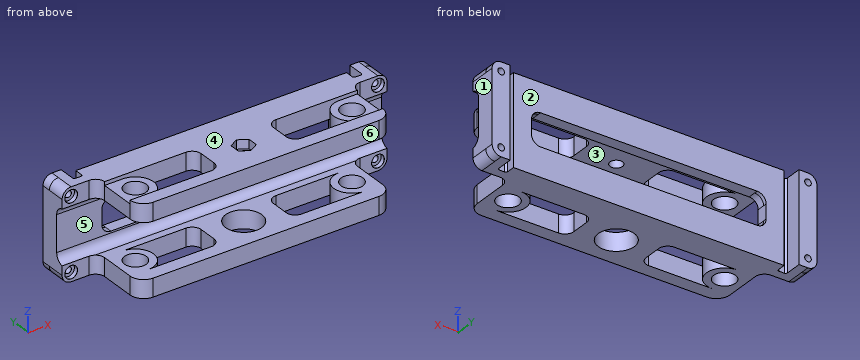
```python
from build123d import *

# Parameters (mm, degrees)
SKETCH_1_W                 = 150
SKETCH_1_H                 = 50
EXTRUDE_1_DEPTH            = 10
CUT_EXTRUDE_5_DEPTH        = 5
SKETCH_6_R                 = 6.05
CUT_EXTRUDE_6_DEPTH        = 80.686887253
CUT_EXTRUDE_7_DEPTH        = 80.686887253
CUT_EXTRUDE_8_DEPTH        = 80.686887253
SKETCH_9_R                 = 3.5
CUT_EXTRUDE_9_DEPTH        = 80.214897721
SKETCH_10_W                = 150
SKETCH_10_H                = 1.5
CUT_EXTRUDE_10_DEPTH       = 80.686887391
SKETCH_11_W                = 150
SKETCH_11_H                = 4.25
EXTRUDE_3_DEPTH            = 15
CUT_EXTRUDE_12_REACH       = 95.152
SKETCH_14_R                = 10
SKETCH_15_W                = 130
SKETCH_15_H                = 18
CUT_EXTRUDE_13_DEPTH       = 93.604333216
FILLET_1_R                 = 5
EXTRUDE_4_DEPTH            = 15
EXTRUDE_5_DEPTH            = 15
FILLET_2_R                 = 5
HOLE_WIZARD_M31_AT_2_COUNT = 2
HOLE_WIZARD_M31_AT_2_PITCH = 40
HOLE_WIZARD_M31_AT_3_COUNT = 2
HOLE_WIZARD_M31_AT_3_PITCH = 170
HOLE_WIZARD_M31_AT_4_COUNT = 2
HOLE_WIZARD_M31_AT_4_PITCH = 174.642491966
CUT_EXTRUDE_20_DEPTH       = 2
SKETCH_22_W                = 5
SKETCH_22_H                = 50
CUT_EXTRUDE_21_DEPTH       = 5
FILLET_3_R                 = 1
FILLET_4_R                 = 5
EXTRUDE_START              = 5
SKETCH_23_R                = 1.825
EXTRUDE_7_DEPTH            = 5
EXTRUDE_START_2            = 2
SKETCH_24_W                = 150
SKETCH_24_H                = 50
EXTRUDE_8_DEPTH            = 2


with BuildPart() as part:
    # Эскиз1 → Бобышка-Вытянуть1 (new body)
    with BuildSketch(Plane.XY):
        Rectangle(SKETCH_1_W, SKETCH_1_H)
    extrude(amount=EXTRUDE_1_DEPTH)

    # Эскиз5 → Вырез-Вытянуть5 (cut)
    with BuildSketch(Plane.XY.offset(10)):
        Polygon((0, 5.75), (-4.979646072, 2.875), (-4.979646072, -2.875), (0, -5.75), (4.979646072, -2.875), (4.979646072, 2.875), align=None)
    extrude(amount=-CUT_EXTRUDE_5_DEPTH, mode=Mode.SUBTRACT)

    # Эскиз6 → Вырез-Вытянуть6 (cut, through all)
    with BuildSketch(Plane.XY.offset(10)):
        with Locations((-60, 0)):
            Circle(SKETCH_6_R)
        with Locations(Location((60, 0, 0), (0, 0, 180))):
            Circle(SKETCH_6_R)
    extrude(amount=-CUT_EXTRUDE_6_DEPTH, mode=Mode.SUBTRACT)

    # Эскиз7 → Вырез-Вытянуть7 (cut, through all)
    with BuildSketch(Plane.XY.offset(10)):
        with BuildLine():
            Line((65, -25), (75, -25))
            Line((75, -25), (75, -15))
            Line((75, -15), (75, 15))
            ThreePointArc((75, 15), (71.464466094, 13.535533906), (70, 10))
            Line((70, 10), (70, -10))
            ThreePointArc((70, -10), (67.803300859, -15.303300859), (62.5, -17.5))
            Line((62.5, -17.5), (27.5, -17.5))
            Line((27.5, -17.5), (-2.5, -17.5))
            Line((-2.5, -17.5), (-32.5, -17.5))
            Line((-32.5, -17.5), (-62.5, -17.5))
            ThreePointArc((-62.5, -17.5), (-67.803300859, -15.303300859), (-70, -10))
            Line((-70, -10), (-70, 10))
            ThreePointArc((-70, 10), (-71.464466094, 13.535533906), (-75, 15))
            Line((-75, 15), (-75, -15))
            Line((-75, -15), (-75, -25))
            Line((-75, -25), (-65, -25))
            Line((-65, -25), (-25, -25))
            Line((-25, -25), (25, -25))
            Line((25, -25), (65, -25))
        make_face()
    extrude(amount=-CUT_EXTRUDE_7_DEPTH, mode=Mode.SUBTRACT)

    # Эскиз8 → Вырез-Вытянуть8 (cut, through all)
    with BuildSketch(Plane(origin=(0, 0, 0), x_dir=(-1, 0, 0), z_dir=(0, 0, -1))):
        with BuildLine():
            Line((20, -5), (20, 5))
            ThreePointArc((20, 5), (21.464466094, 8.535533906), (25, 10))
            Line((25, 10), (45, 10))
            add(Edge.make_bspline(
                [(60, 10), (59.955521003, 10), (54.127943117, 10), (45, 10)],
                knots=[0, 0, 0, 0, 1, 1, 1, 1], degree=3))
            ThreePointArc((60, 10), (50, 0), (60, -10))
            add(Edge.make_bspline(
                [(60, -10), (59.955521003, -10), (54.127943117, -10), (45, -10)],
                knots=[0, 0, 0, 0, 1, 1, 1, 1], degree=3))
            Line((45, -10), (25, -10))
            ThreePointArc((25, -10), (21.464466094, -8.535533906), (20, -5))
        make_face()
        with BuildLine():
            Line((-45, -10), (-25, -10))
            ThreePointArc((-25, -10), (-21.464466094, -8.535533906), (-20, -5))
            Line((-20, -5), (-20, 5))
            ThreePointArc((-20, 5), (-21.464466094, 8.535533906), (-25, 10))
            Line((-25, 10), (-45, 10))
            add(Edge.make_bspline(
                [(-60, 10), (-59.955521003, 10), (-54.127943117, 10), (-45, 10)],
                knots=[0, 0, 0, 0, 1, 1, 1, 1], degree=3))
            ThreePointArc((-60, 10), (-50, 0), (-60, -10))
            add(Edge.make_bspline(
                [(-60, -10), (-59.955521003, -10), (-54.127943117, -10), (-45, -10)],
                knots=[0, 0, 0, 0, 1, 1, 1, 1], degree=3))
        make_face()
    extrude(amount=-CUT_EXTRUDE_8_DEPTH, mode=Mode.SUBTRACT)

    # Эскиз9 → Вырез-Вытянуть9 (cut, through all)
    with BuildSketch(Plane.XY.offset(5)):
        Circle(SKETCH_9_R)
    extrude(amount=-CUT_EXTRUDE_9_DEPTH, mode=Mode.SUBTRACT)

    # Эскиз10 → Вырез-Вытянуть10 (cut, through all)
    with BuildSketch(Plane.XY.offset(10)):
        with Locations((0, 24.25)):
            Rectangle(SKETCH_10_W, SKETCH_10_H)
    extrude(amount=-CUT_EXTRUDE_10_DEPTH, mode=Mode.SUBTRACT)

    # Эскиз11 → Бобышка-Вытянуть3 (add)
    with BuildSketch(Plane(origin=(0, 0, 0), x_dir=(-1, 0, 0), z_dir=(0, 0, -1))):
        with Locations((0, 21.375)):
            Rectangle(SKETCH_11_W, SKETCH_11_H)
    extrude(amount=EXTRUDE_3_DEPTH)

    # Зеркальное отражение9: part across plane


with BuildPart() as part_1:
    add(part.part)
    add(part.part.mirror(Plane(origin=(0, 0, -15), x_dir=(1, 0, 0), z_dir=(0, 0, -1))))

    # Эскиз14 → Вырез-Вытянуть12 (cut, up to next)
    with BuildSketch(Plane(origin=(0, 0, -40), x_dir=(-1, 0, 0), z_dir=(0, 0, -1)), mode=Mode.PRIVATE) as cut_extrude_12_sk1:
        Circle(SKETCH_14_R)
    cut_extrude_12_tool1 = extrude(cut_extrude_12_sk1.sketch, amount=-CUT_EXTRUDE_12_REACH, mode=Mode.PRIVATE) & part_1.part
    add(cut_extrude_12_tool1.solids().sort_by_distance((0, 0, -40))[0], mode=Mode.SUBTRACT)

    # Эскиз15 → Вырез-Вытянуть13 (cut, through all)
    with BuildSketch(Plane.XZ.offset(-19.25)):
        with Locations((0, -15)):
            Rectangle(SKETCH_15_W, SKETCH_15_H)
    extrude(amount=-CUT_EXTRUDE_13_DEPTH, mode=Mode.SUBTRACT)

    # Скругление1
    fillet_1_edges = [part_1.edges().sort_by_distance(p)[0] for p in [
        (65, 21.375, -6),
        (65, 21.375, -24),
        (-65, 21.375, -24),
        (-65, 21.375, -6),
    ]]
    fillet(fillet_1_edges, radius=FILLET_1_R)

    # Эскиз18 → Бобышка-Вытянуть4 (add)
    with BuildSketch(Plane(origin=(75, 0, 0), x_dir=(0, 0, -1), z_dir=(1, 0, 0))):
        Polygon((-10, 23.5), (-10, 15), (0, 15), (0, 19.25), (30, 19.25), (30, 15), (40, 15), (40, 25), (-10, 25), align=None)
    extrude(amount=EXTRUDE_4_DEPTH)

    # Эскиз19 → Бобышка-Вытянуть5 (add)
    with BuildSketch(Plane.ZY.offset(75)):
        Polygon((-40, 15), (-30, 15), (-30, 19.25), (0, 19.25), (0, 15), (10, 15), (10, 25), (-40, 25), align=None)
    extrude(amount=EXTRUDE_5_DEPTH)

    # Скругление2
    fillet_2_edges = [part_1.edges().sort_by_distance(p)[0] for p in [
        (90, 20, 10),
        (90, 20, -40),
        (-90, 20, -40),
        (-90, 20, 10),
    ]]
    fillet(fillet_2_edges, radius=FILLET_2_R)

    # Эскиз20 → Цековка для винта с заклепочной головкой M31 (revolve, cut)
    with BuildSketch(Plane(origin=(-85, 15, -35), x_dir=(0, 0, -1), z_dir=(1, 0, 0))):
        Polygon((0, 0), (0, 10), (1.825, 10), (1.8, 9.975), (1.8, 2.425), (1.825, 2.4), (3.5, 2.4), (3.5, 0.025), (3.525, 0), align=None)
    hole_wizard_m31 = revolve(axis=Axis((-85, 8.65, -35), (0, 1, 0)), mode=Mode.SUBTRACT)

    # Цековка для винта с заклепочной головкой M31 at 2: Цековка для винта с заклепочной головкой M31 ×2
    with Locations(*[(0, 0, i * HOLE_WIZARD_M31_AT_2_PITCH) for i in range(1, HOLE_WIZARD_M31_AT_2_COUNT)]):
        add(hole_wizard_m31, mode=Mode.SUBTRACT)

    # Цековка для винта с заклепочной головкой M31 at 3: Цековка для винта с заклепочной головкой M31 ×2
    with Locations(*[(i * HOLE_WIZARD_M31_AT_3_PITCH, 0, 0) for i in range(1, HOLE_WIZARD_M31_AT_3_COUNT)]):
        add(hole_wizard_m31, mode=Mode.SUBTRACT)

    # Цековка для винта с заклепочной головкой M31 at 4: Цековка для винта с заклепочной головкой M31 ×2
    with Locations(*[Vector(0.9734171683335759, 0, 0.2290393337255473) * (i * HOLE_WIZARD_M31_AT_4_PITCH) for i in range(1, HOLE_WIZARD_M31_AT_4_COUNT)]):
        add(hole_wizard_m31, mode=Mode.SUBTRACT)

    # Эскиз21 → Вырез-Вытянуть20 (cut)
    with BuildSketch(Plane.XY.offset(10)):
        with BuildLine():
            Line((-60, 10), (-70, 10))
            Line((-70, 10), (-70, -10))
            Line((-70, -10), (-60, -10))
            ThreePointArc((-60, -10), (-50, 0), (-60, 10))
        make_face()
        with BuildLine():
            Line((60, 10), (70, 10))
            Line((70, 10), (70, -10))
            Line((70, -10), (60, -10))
            ThreePointArc((60, -10), (50, 0), (60, 10))
        make_face()
    extrude(amount=-CUT_EXTRUDE_20_DEPTH, mode=Mode.SUBTRACT)

    # Эскиз22 → Вырез-Вытянуть21 (cut)
    with BuildSketch(Plane(origin=(0, 25, 0), x_dir=(1, 0, 0), z_dir=(0, 1, 0))):
        with Locations((77.5, 15)):
            Rectangle(SKETCH_22_W, SKETCH_22_H)
        with Locations((-77.5, 15)):
            Rectangle(SKETCH_22_W, SKETCH_22_H)
    extrude(amount=-CUT_EXTRUDE_21_DEPTH, mode=Mode.SUBTRACT)

    # Скругление3
    fillet_3_edges = [part_1.edges().sort_by_distance(p)[0] for p in [
        (75, 20, -15),
        (80, 20, -15),
        (-75, 20, -15),
        (-80, 20, -15),
    ]]
    fillet(fillet_3_edges, radius=FILLET_3_R)

    # Скругление4
    fillet_4_edges = [part_1.edges().sort_by_distance(p)[0] for p in [
        (0, 19.25, 0),
        (0, 19.25, -30),
    ]]
    fillet(fillet_4_edges, radius=FILLET_4_R)

    # Эскиз23 → Бобышка-Вытянуть7 (add)
    # profile 1 of 2: a face of its own
    with BuildSketch(Plane(origin=(0, 25, 0), x_dir=(1, 0, 0), z_dir=(0, 1, 0)).offset(EXTRUDE_START)):
        with BuildLine():
            Line((-80, 40), (-80, -10))
            Line((-80, -10), (-85, -10))
            ThreePointArc((-85, -10), (-88.535533906, -8.535533906), (-90, -5))
            Line((-90, -5), (-90, 35))
            ThreePointArc((-90, 35), (-88.535533906, 38.535533906), (-85, 40))
            Line((-85, 40), (-80, 40))
        make_face()
        with Locations(Location((-85, 35, 0), (0, 0, 90))):
            Circle(SKETCH_23_R, mode=Mode.SUBTRACT)
        with Locations(Location((-85, -5, 0), (0, 0, 90))):
            Circle(SKETCH_23_R, mode=Mode.SUBTRACT)
    # profile 2 of 2: a face of its own
    with BuildSketch(Plane(origin=(0, 25, 0), x_dir=(1, 0, 0), z_dir=(0, 1, 0)).offset(EXTRUDE_START)):
        with BuildLine():
            Line((80, 40), (80, -10))
            Line((80, -10), (85, -10))
            ThreePointArc((85, -10), (88.535533906, -8.535533906), (90, -5))
            Line((90, -5), (90, 35))
            ThreePointArc((90, 35), (88.535533906, 38.535533906), (85, 40))
            Line((85, 40), (80, 40))
        make_face()
        with Locations(Location((85, 35, 0), (0, 0, 90))):
            Circle(SKETCH_23_R, mode=Mode.SUBTRACT)
        with Locations(Location((85, -5, 0), (0, 0, 90))):
            Circle(SKETCH_23_R, mode=Mode.SUBTRACT)
    extrude(amount=-EXTRUDE_7_DEPTH)

    # Эскиз24 → Бобышка-Вытянуть8 (add)
    with BuildSketch(Plane(origin=(0, 23.5, 0), x_dir=(1, 0, 0), z_dir=(0, 1, 0)).offset(EXTRUDE_START_2)):
        with Locations((0, 15)):
            Rectangle(SKETCH_24_W, SKETCH_24_H)
        with BuildLine():
            Line((-60, 24), (60, 24))
            ThreePointArc((60, 24), (63.535533906, 22.535533906), (65, 19))
            Line((65, 19), (65, 11))
            ThreePointArc((65, 11), (63.535533906, 7.464466094), (60, 6))
            Line((60, 6), (-60, 6))
            ThreePointArc((-60, 6), (-63.535533906, 7.464466094), (-65, 11))
            Line((-65, 11), (-65, 19))
            ThreePointArc((-65, 19), (-63.535533906, 22.535533906), (-60, 24))
        make_face(mode=Mode.SUBTRACT)
    extrude(amount=-EXTRUDE_8_DEPTH)


solid = part_1.part
```
Build history of the part. All positions in model axes, mm. Face numbers are marked on the shaded views. A direction names the side the tool comes from. Round coordinates to 2 decimals unless told otherwise and drop trailing zeros. Order: outer loops, then holes, each group sorted by start corner. A loop starts at its lowest first (then second) coordinate and runs counter-clockwise, first axis right, second up. Notation, with made-up numbers: (0.25, -29.5) -> (50.25, -29.5) arc R17 ccw to (50.25, -3.5) -> close; hole circle Ø11 at (35, -16). An arc over 180 degrees is marked (long way). Answer in a Markdown table with one row per item.
1) Band-saw the part on A-A on x = -27. Give the cut face in (y, z), and give its area (3 significant figures).
Values:
| item | result |
|---|---|
| outline | (-17.5, -40) -> (-10, -40) -> (-10, -30) -> (-17.5, -30) -> close; (-17.5, 0) -> (-10, 0) -> (-10, 10) -> (-17.5, 10) -> close; (10, -40) -> (25.5, -40) -> (25.5, -24) -> (19.25, -24) -> (19.25, -25) arc R5 cw to (14.25, -30) -> (10, -30) -> close; (10, 0) -> (14.25, 0) arc R5 cw to (19.25, -5) -> (19.25, -6) -> (25.5, -6) -> (25.5, 10) -> (10, 10) -> close |
| area | 546 mm2 |
2) Band-saw the part on B-B on z = -15. Give the cut face in (x, y), and give its area (3 significant figures).
Values:
| item | result |
|---|---|
| outline | (-90, 19.25) -> (-65, 19.25) -> (-65, 25.5) -> (-75, 25.5) -> (-75, 21) arc R1 cw to (-76, 20) -> (-79, 20) arc R1 cw to (-80, 21) -> (-80, 30) -> (-90, 30) -> close; (65, 19.25) -> (90, 19.25) -> (90, 30) -> (80, 30) -> (80, 21) arc R1 cw to (79, 20) -> (76, 20) arc R1 cw to (75, 21) -> (75, 25.5) -> (65, 25.5) -> close |
| area | 348 mm2 |
3) Which spindle directions (+Z, -Z, +X, -X, +Y, -Y) get a long thin tool onto all of the face, cutting with end or side? Do the marked faces 1, 2 and 3. Say none if no direction does.
Values:
| item | result |
|---|---|
| face 1 | +Z, -Z, +X, +Y, -Y |
| face 2 | +Z, -Z, +Y |
| face 3 | +X, -X, -Y |
4) Wall check: L1, parallel to X at y = 17, z = -32; L2, parallel to X at y = 25, z = -3.5; L3, parallel to Z at x = -61.5, y = -9.5. Give the ranges that are in metal, low to high.
Values:
| item | result |
|---|---|
| L1 | -90 to -86.8, -83.2 to 83.2, 86.8 to 90 |
| L2 | -90 to -80, -75 to 75, 80 to 90 |
| L3 | -40 to -30, 0 to 8 |
5) Pin check, flat tips, straight feed: P1, Ø8, axis at x = -13, z = -11.5, coming from the -Y side; P2, Ø4, axis at x = 85, z = -35, coming from the -Y side; P3, Ø10, axis at x = 48.5, z = -6.5, coming from the -Y side; P4, Ø6.5, axis at y = -2.5, z = 5, coming from the -X side. Stop position of each tip, or through.
Values:
| item | result |
|---|---|
| P1 | through |
| P2 | y = 17.4 |
| P3 | y = 17.82 |
| P4 | x = -70 |
6) Band-saw the part on C-C on y = 0. Give the number of separate pieces and of enclosed holes in the cut face, and give its area (3 significant figures).
Values:
| item | result |
|---|---|
| separate pieces | 12 |
| enclosed holes | 0 |
| area | 800 mm2 |
7) Mould opens along Z. For the marked faces 4, 5 and 6 say: released by +Z, released by -Z, zero draft, split by the parting line, or undercut.
Values:
| item | result |
|---|---|
| face 4 | released by +Z |
| face 5 | undercut |
| face 6 | zero draft |
